Verification items for the finished model (mm, model axes). A direction names the side the tool comes from. Round coordinates to 2 decimals unless told otherwise and drop trailing zeros. Order: outer loops, then holes, each group sorted by start corner. A loop starts at its lowest first (then second) coordinate and runs counter-clockwise, first axis right, second up. Notation, with made-up numbers: (54.5, 69.5) -> (76.5, 69.5) arc R25 cw to (76.5, 103.5) -> close; hole circle Ø10 at (42.5, 36.25). An arc over 180 degrees is marked (long way). Write item = value, one per line. Start each with the question number.
from build123d import *

# Parameters (mm, degrees)
SKETCH1_W           = 25
SKETCH1_H           = 25
BOSS_EXTRUDE1_DEPTH = 25
SHELL1_T            = 2.5
SKETCH2_W           = 12
SKETCH2_H           = 12
CUT_EXTRUDE1_DEPTH  = 15
SKETCH3_R           = 2.5
CUT_EXTRUDE2_DEPTH  = 15
SKETCH4_R           = 2.5
CUT_EXTRUDE6_DEPTH  = 15
SKETCH4_3_R         = 2.5
CUT_EXTRUDE7_DEPTH  = 15
SKETCH5_R           = 2.5
CUT_EXTRUDE8_DEPTH  = 15
SKETCH5_4_R         = 2.5
CUT_EXTRUDE9_DEPTH  = 15
SKETCH5_5_R         = 2.5
CUT_EXTRUDE10_DEPTH = 15
SKETCH7_R           = 2.5
CUT_EXTRUDE11_DEPTH = 15
SKETCH8_R           = 2.5
CUT_EXTRUDE12_DEPTH = 10


with BuildPart() as part:
    # Sketch1 → Boss-Extrude1 (new body)
    with BuildSketch(Plane(origin=(0, 0, 0), x_dir=(1, 0, 0), z_dir=(0, 1, 0))):
        Rectangle(SKETCH1_W, SKETCH1_H)
    extrude(amount=BOSS_EXTRUDE1_DEPTH)

    # Shell1 (no face opened: a closed hollow body)
    add(offset(amount=-SHELL1_T, mode=Mode.PRIVATE), mode=Mode.SUBTRACT)

    # Sketch2 → Cut-Extrude1 (cut)
    with BuildSketch(Plane(origin=(0, 25, 0), x_dir=(1, 0, 0), z_dir=(0, 1, 0))):
        Rectangle(SKETCH2_W, SKETCH2_H)
    extrude(amount=-CUT_EXTRUDE1_DEPTH, mode=Mode.SUBTRACT)

    # Sketch3 → Cut-Extrude2 (cut)
    with BuildSketch(Plane.XZ):
        with Locations((-5, 7)):
            Circle(SKETCH3_R)
        with Locations((-5, 0)):
            Circle(SKETCH3_R)
        with Locations((-5, -7)):
            Circle(SKETCH3_R)
        with Locations((5, 7)):
            Circle(SKETCH3_R)
        with Locations((5, 0)):
            Circle(SKETCH3_R)
        with Locations((5, -7)):
            Circle(SKETCH3_R)
    extrude(amount=-CUT_EXTRUDE2_DEPTH, mode=Mode.SUBTRACT)

    # Sketch4 → Cut-Extrude6 (cut)
    with BuildSketch(Plane(origin=(12.5, 0, 0), x_dir=(0, 0, -1), z_dir=(1, 0, 0))):
        with Locations((-5, 17.5)):
            Circle(SKETCH4_R)
    extrude(amount=-CUT_EXTRUDE6_DEPTH, mode=Mode.SUBTRACT)

    # Sketch4<3> → Cut-Extrude7 (cut)
    with BuildSketch(Plane(origin=(12.5, 0, 0), x_dir=(0, 0, -1), z_dir=(1, 0, 0))):
        with Locations((0, 12.5)):
            Circle(SKETCH4_3_R)
        with Locations((5, 7.5)):
            Circle(SKETCH4_3_R)
    extrude(amount=-CUT_EXTRUDE7_DEPTH, mode=Mode.SUBTRACT)

    # Sketch5 → Cut-Extrude8 (cut)
    with BuildSketch(Plane.ZY.offset(12.5)):
        with Locations((-6, 18.5)):
            Circle(SKETCH5_R)
    extrude(amount=-CUT_EXTRUDE8_DEPTH, mode=Mode.SUBTRACT)

    # Sketch5<4> → Cut-Extrude9 (cut)
    with BuildSketch(Plane.ZY.offset(12.5)):
        with Locations((6, 18.5)):
            Circle(SKETCH5_4_R)
    extrude(amount=-CUT_EXTRUDE9_DEPTH, mode=Mode.SUBTRACT)

    # Sketch5<5> → Cut-Extrude10 (cut)
    with BuildSketch(Plane.ZY.offset(12.5)):
        with Locations((6, 6.5)):
            Circle(SKETCH5_5_R)
        with Locations((-6, 6.5)):
            Circle(SKETCH5_5_R)
    extrude(amount=-CUT_EXTRUDE10_DEPTH, mode=Mode.SUBTRACT)

    # Sketch7 → Cut-Extrude11 (cut)
    with BuildSketch(Plane.XY.offset(12.5)):
        with Locations((-6, 18.5)):
            Circle(SKETCH7_R)
        with Locations((0, 12.5)):
            Circle(SKETCH7_R)
        with Locations((6, 18.5)):
            Circle(SKETCH7_R)
        with Locations((6, 6.5)):
            Circle(SKETCH7_R)
        with Locations((-6, 6.5)):
            Circle(SKETCH7_R)
    extrude(amount=-CUT_EXTRUDE11_DEPTH, mode=Mode.SUBTRACT)

    # Sketch8 → Cut-Extrude12 (cut)
    with BuildSketch(Plane(origin=(0, 0, -12.5), x_dir=(-1, 0, 0), z_dir=(0, 0, -1))):
        with Locations((0, 18.5)):
            Circle(SKETCH8_R)
        with Locations((0, 6.5)):
            Circle(SKETCH8_R)
    extrude(amount=-CUT_EXTRUDE12_DEPTH, mode=Mode.SUBTRACT)


solid = part.part
(1) Cross-section at D-D (z = 1). Enter the section's corners in (x, y).
(2) Draft check along Y on faces 5 (the cylindrical face through (11.27, 5.28, -6.15)), 6 (the cylindrical face through (7.31, 1.23, -7.96)). Enter one of: +Y half, -Y half, draft (parallel to the pull), parting line (faces both ways), or undercut.
(3) Scan lines: line 1 along Z through (x, y) = (-5, 1.05); line 2 along Y through (x, z) = (-11.5, -6); line 3 along Z through (x, y) = (-1, 21.25). Record each from-to range of solid material in increasing order. Write a range as from..to.
(4) Set-up check for faces 1 (the flat face through (0, 22.5, -7)), 2 (the flat face through (-6, 24, 0)), 3 (the cylindrical face through (-11.27, 20.61, 7.34)), 4 (the cylindrical face through (-2.69, 1.23, -7.96)): record each of +Z, -Z, +X, -X, +Y, -Y from which the full face is reachable in a straight line by a thin tool's end or side.
(5) Cross-section at C-C (y = 10.5). Enter the section's corners in (x, z), and give its area (3 significant figures).
(6) Cross-section at B-B (x = 9.5). Enter the section's corners in (y, z).
(7) Cross-section at A-A (y = 4.5). Enter the section's corners in (x, z), and give its area (4 significant figures).
(8) Depth check by flat-ended pin: pin 1 (3 mm diameter, centred on x = -5, z = 7, fed in from -Y); pin 2 (3 mm diameter, centred on y = 6.5, z = 6, fed in from -X); pin 3 (1 mm diameter, centred on x = 0, z = -4.5, fed in from +Y). Enter the tip coordinate at first touch or a pass-through.
Outcome:
q1.outline = (-12.5, 0) -> (-7.29, 0) -> (-7.29, 2.5) -> (-10, 2.5) -> (-10, 22.5) -> (-6, 22.5) -> (-6, 25) -> (-12.5, 25) -> close; (-2.71, 0) -> (2.71, 0) -> (2.71, 2.5) -> (-2.71, 2.5) -> close; (6, 22.5) -> (10, 22.5) -> (10, 14.79) -> (12.5, 14.79) -> (12.5, 25) -> (6, 25) -> close; (7.29, 0) -> (12.5, 0) -> (12.5, 10.21) -> (10, 10.21) -> (10, 2.5) -> (7.29, 2.5) -> close
q2.face_5 = undercut
q2.face_6 = draft
q3.line_1 = -12.5..-9.5, -4.5..-2.5, 2.5..4.5, 9.5..12.5
q3.line_2 = 0..4, 9..16, 21..25
q3.line_3 = -12.5..-10, 10..12.5
q4.face_1 = none
q4.face_2 = +Y
q4.face_3 = -X
q4.face_4 = -Y
q5.outline = (-12.5, -12.5) -> (12.5, -12.5) -> (12.5, -1.5) -> (10, -1.5) -> (10, -10) -> (-10, -10) -> (-10, 10) -> (-1.5, 10) -> (-1.5, 12.5) -> (-12.5, 12.5) -> close; (1.5, 10) -> (10, 10) -> (10, 1.5) -> (12.5, 1.5) -> (12.5, 12.5) -> (1.5, 12.5) -> close
q5.area = 210 mm^2
q6.outline = (0, -12.5) -> (25, -12.5) -> (25, 12.5) -> (0, 12.5) -> close; hole (2.5, -10) -> (22.5, -10) -> (22.5, 10) -> (2.5, 10) -> close
q7.outline = (-12.5, -12.5) -> (-1.5, -12.5) -> (-1.5, -10) -> (-10, -10) -> (-10, -7.5) -> (-12.5, -7.5) -> close; (-12.5, -4.5) -> (-10, -4.5) -> (-10, 4.5) -> (-12.5, 4.5) -> close; (-12.5, 7.5) -> (-10, 7.5) -> (-10, 10) -> (-7.5, 10) -> (-7.5, 12.5) -> (-12.5, 12.5) -> close; (-4.5, 10) -> (4.5, 10) -> (4.5, 12.5) -> (-4.5, 12.5) -> close; (1.5, -12.5) -> (12.5, -12.5) -> (12.5, 12.5) -> (7.5, 12.5) -> (7.5, 10) -> (10, 10) -> (10, -10) -> (1.5, -10) -> close
q7.area = 187.5 mm^2
q8.pin_1 = 22.5
q8.pin_2 = 10
q8.pin_3 = 2.5
